The model under review builds one solid part; all positions refer to its coordinate system, in mm. A direction names the side the tool comes from. Coordinates: 2 decimals unless noted, no trailing zeros. Loops run counter-clockwise (first coordinate to the right, second up) from the corner with the lowest first, then second, coordinate; pieces in that order, holes last. Notation, with made-up numbers: (-38, 34.25) - (-27, 34.25) arc R35 ccw to (-27, 71.25) - close; hole circle Ø6 at (89.5, -8). An arc over 180 degrees is marked (long way). Use a Markdown table: item, result. Add a question column.
1) For faces 1 (the flat face through (22.225, 17, 18)), 2 (the flat face through (47, 25.4, 42)), 3 (the flat face through (87, 0, 38.1)), list the 3-axis set-ups (+Z, -Z, +X, -X, +Y, -Y) from which the entire face can be reached by the end or side of a thin tool; tool diameter is ignored.
2) The part is to be moulded in two halves that separate along X. For faces 4 (the conical face through (64.54, -0.97, 66.55)), 5 (the flat face through (-2, 7.938, 32)), 6 (the flat face through (61.9, -0.4, 42.875)), say which applies: pulls with the +X half, pulls with the -X half, needs draft (parallel to the pull), parting line crosses it, or undercut.
3) To check wall thickness, follow L1, parallel to Z at x = -13.5, y = 36.5 (3 decimals); L2, parallel to Y at x = 20, z = 23.5; L3, parallel to X at y = -45.5, z = -1 (3 decimals). State the ranges of each line that lie inside material, in increasing order. Write a range as [from, to].
4) Clearance check with flat-ended pins moving along their axes: pin 1 (1.5 mm diameter, centred on y = 5.5, z = 17, fed in from +X) (3 decimals); pin 2 (14 mm diameter, centred on y = 13, z = 20.5, fed in from -X); pin 3 (5 mm diameter, centred on x = 8.5, y = -24, fed in from +Z) (3 decimals). State where each tip first meets the part, or that it passes through.
5) Add section A-A, the plane z = 7. Give the boundary of the cut face in (x, y) (3 decimals).
6) Add section B-B, the plane y = -44. Give the boundary of the cut face in (x, z) (3 decimals).
```python
from build123d import *

# Parameters (mm, degrees)
F1_DEPTH = 63.5
F2_DEPTH = 25.4
F3_DEPTH = 7.9375
F5_R     = 6.35
F6_SIZE  = 2.54


with BuildPart() as f1:
    # F0 (on Front) → F1 (new body, symmetric)
    with BuildSketch(Plane.XZ):
        Polygon((22.225, 9.525), (-41.275, 9.525), (-41.275, -9.525), (41.275, -9.525), (41.275, 9.525), align=None)
    extrude(amount=F1_DEPTH, both=True)

    # F0 (on Front) → F2 (join, symmetric)
    with BuildSketch(Plane.XZ):
        with BuildLine():
            Line((22.225, 27.0002), (22.225, 9.525))
            Line((22.225, 9.525), (41.275, 9.525))
            Line((41.275, 9.525), (41.275, 27.0002))
            ThreePointArc((41.275, 27.0002), (45.9246798487, 38.2255201513), (57.15, 42.8752))
            Line((57.15, 42.8752), (60.325, 42.8752))
            Line((60.325, 42.8752), (60.325, 61.9252))
            Line((60.325, 61.9252), (57.15, 61.9252))
            ThreePointArc((57.15, 61.9252), (32.4542956671, 51.6959043329), (22.225, 27.0002))
        make_face()
        Polygon((86.6135649812, 61.9252), (60.325, 61.9252), (60.325, 42.8752), (76.2353741971, 42.8752), (86.6135649812, 42.8752), align=None)
    extrude(amount=F2_DEPTH, both=True)

    # F0 (on Front) → F3 (join, symmetric)
    with BuildSketch(Plane.XZ):
        with BuildLine():
            add(Edge.make_bspline(
                [(-41.275, 9.525), (-41.1990918219, 33.1209041178), (17.5218340009, 65.2216747403), (57.15, 61.9252)],
                knots=[0, 0, 0, 0, 111.5045361635, 111.5045361635, 111.5045361635, 111.5045361635], degree=3))
            Line((-41.275, 9.525), (22.225, 9.525))
            Line((22.225, 9.525), (22.225, 27.0002))
            ThreePointArc((22.225, 27.0002), (32.4542956671, 51.6959043329), (57.15, 61.9252))
        make_face()
    extrude(amount=F3_DEPTH, both=True)

    # F0 (on Front) → F4 (revolve)
    with BuildSketch(Plane.XZ):
        Polygon((86.6135649812, 66.675), (86.6135649812, 61.9252), (86.6135649812, 42.8752), (86.6135649812, 38.1), (111.125, 38.1), (111.125, 66.675), align=None)
    revolve(axis=Axis((86.6135649812, 0, 52.3875), (0, 0, -1)))

    # F5
    f5_edges = [f1.edges().sort_by_distance(p)[0] for p in [
        (-41.275, -63.5, 0),
        (41.275, -63.5, 0),
        (41.275, 63.5, 0),
        (-41.275, 63.5, 0),
    ]]
    fillet(f5_edges, radius=F5_R)

    # F6
    f6_edges = [f1.edges().sort_by_distance(p)[0] for p in [
        (62.10213, 0, 66.675),
    ]]
    chamfer(f6_edges, length=F6_SIZE)


solid = f1.part
```
From the geometry:
| question | item | result |
|---|---|---|
| 1 | face 1 | +Z, -X, +Y |
| 1 | face 2 | +Z, +X, -X, +Y |
| 1 | face 3 | -Z, +X, +Y, -Y |
| 2 | face 4 | parting line crosses it |
| 2 | face 5 | needs draft |
| 2 | face 6 | undercut |
| 3 | L1 | z = [-9.525, 9.525] |
| 3 | L2 | y = [-7.94, 7.94] |
| 3 | L3 | x = [-41.275, 41.275] |
| 4 | pin 1 | stops at x = 41.275 |
| 4 | pin 2 | stops at x = -40.05 |
| 4 | pin 3 | stops at z = 9.525 |
| 5 | outline | (-41.275, -57.15) arc R6.35 ccw to (-34.925, -63.5) - (34.925, -63.5) arc R6.35 ccw to (41.275, -57.15) - (41.275, 57.15) arc R6.35 ccw to (34.925, 63.5) - (-34.925, 63.5) arc R6.35 ccw to (-41.275, 57.15) - close |
| 6 | outline | (-41.275, -9.525) - (41.275, -9.525) - (41.275, 9.525) - (-41.275, 9.525) - close |
